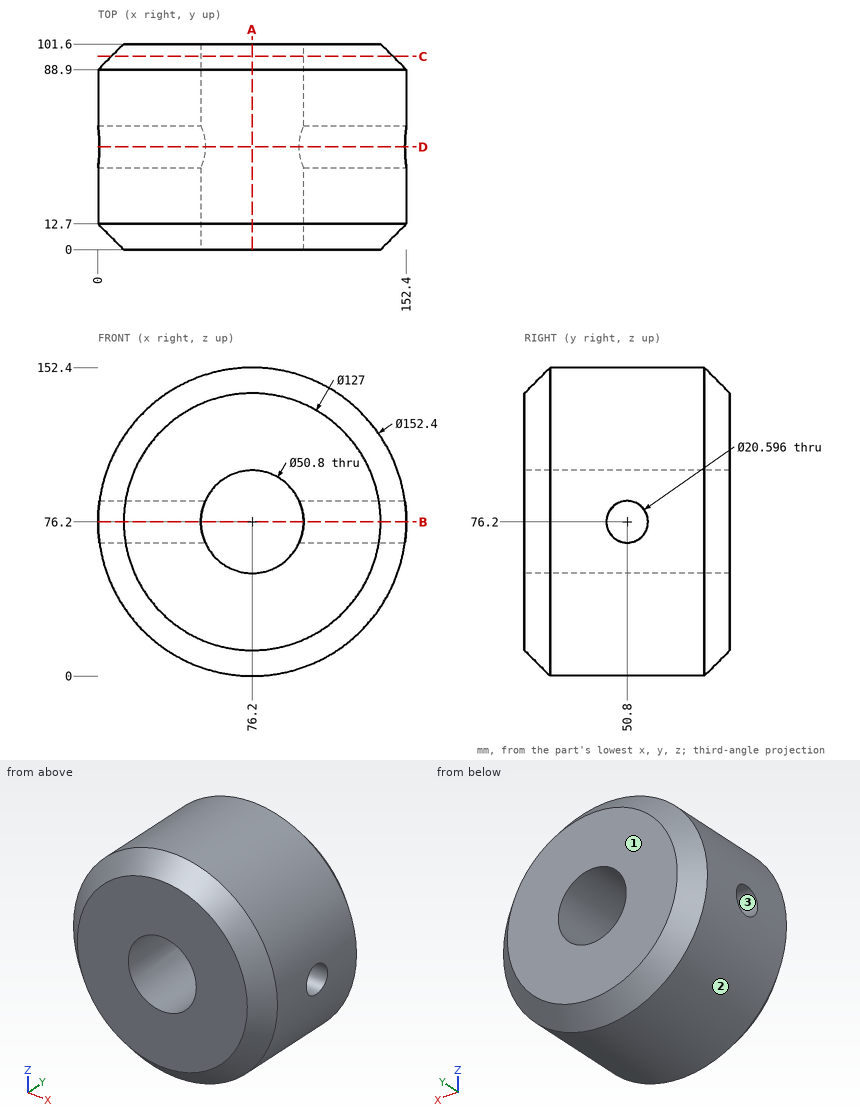
Study the drawing (mm; zero at the part's minimum x, y, z) and answer. Coordinates: 2 decimals unless noted, no trailing zeros. Loops run counter-clockwise (first coordinate to the right, second up) from the corner with the lowest first, then second, coordinate; pieces in that order, holes last. Notation, with made-up numbers: (4.5, 19.25) -> (40.5, 19.25) arc R11 ccw to (40.5, 29.25) -> close; hole circle Ø1 at (-11, 77.5). An arc over 180 degrees is marked (long way). Answer in a Markdown table with one row per item. Add a question column.
1. Flat-ended cylindrical pins translate along their axes: P1, Ø6, axis at y = 51.5, z = 29, coming from the -X side; P2, Ø10, axis at x = 111, y = 71, coming from the +Z side; P3, Ø1, axis at x = 25.5, y = 34.5, coming from the -Z side. Find the tip coordinate at first contact, or state that the pin passes through.
2. The part is cut by section C-C, the plane y = 95.5. Write down the section's boundary in (x, z).
3. Determine the mould class of the marked faces 1, 2 and 3 for opening direction Z: +Z half, -Z half, draft (parallel to the pull), parting line (faces both ways), or undercut.
4. The part is cut by section A-A, the plane x = 76.2. Write down the section's boundary in (y, z), then the cut area to 4 significant figures.
5. Consider line 1 (Z direction, x = 76.2, y = 49.5); line 2 (X direction, y = 37, z = 75); line 3 (Z direction, x = 134, y = 57) (1 decimal). Determine where each line is inside the solid, lowest interval first. Write a range as [from, to].
6. The part is cut by section D-D, the plane y = 50.8. Write down the section's boundary in (x, z).
7. The part is cut by section B-B, the plane z = 76.2. Write down the section's boundary in (x, y).
Answer below:
| question | item | result |
|---|---|---|
| 1 | P1 | x = 14.13 |
| 1 | P2 | z = 146.33 |
| 1 | P3 | z = 18.87 |
| 2 | outline | circle Ø139.2 at (76.2, 76.2); hole circle Ø50.8 at (76.2, 76.2) |
| 3 | face 1 | draft |
| 3 | face 2 | parting line |
| 3 | face 3 | undercut |
| 4 | outline | (0, 12.7) -> (12.7, 0) -> (88.9, 0) -> (101.6, 12.7) -> (101.6, 50.8) -> (0, 50.8) -> close; (0, 101.6) -> (101.6, 101.6) -> (101.6, 139.7) -> (88.9, 152.4) -> (12.7, 152.4) -> (0, 139.7) -> close |
| 4 | area | 10,000 mm2 |
| 5 | line 1 | [0, 50.8], [101.6, 152.4] |
| 5 | line 2 | [0.01, 50.83], [101.57, 152.39] |
| 5 | line 3 | [26.5, 68], [84.4, 125.9] |
| 6 | outline | (0.7, 65.9) arc R76.2 ccw to (151.7, 65.9) -> (99.42, 65.9) arc R25.4 cw to (52.98, 65.9) -> close; (0.7, 86.5) -> (52.98, 86.5) arc R25.4 cw to (99.42, 86.5) -> (151.7, 86.5) arc R76.2 ccw to start |
| 7 | outline | (0, 12.7) -> (12.7, 0) -> (50.8, 0) -> (50.8, 40.5) -> (0, 40.5) -> close; (0, 61.1) -> (50.8, 61.1) -> (50.8, 101.6) -> (12.7, 101.6) -> (0, 88.9) -> close; (101.6, 0) -> (139.7, 0) -> (152.4, 12.7) -> (152.4, 40.5) -> (101.6, 40.5) -> close; (101.6, 61.1) -> (152.4, 61.1) -> (152.4, 88.9) -> (139.7, 101.6) -> (101.6, 101.6) -> close |
